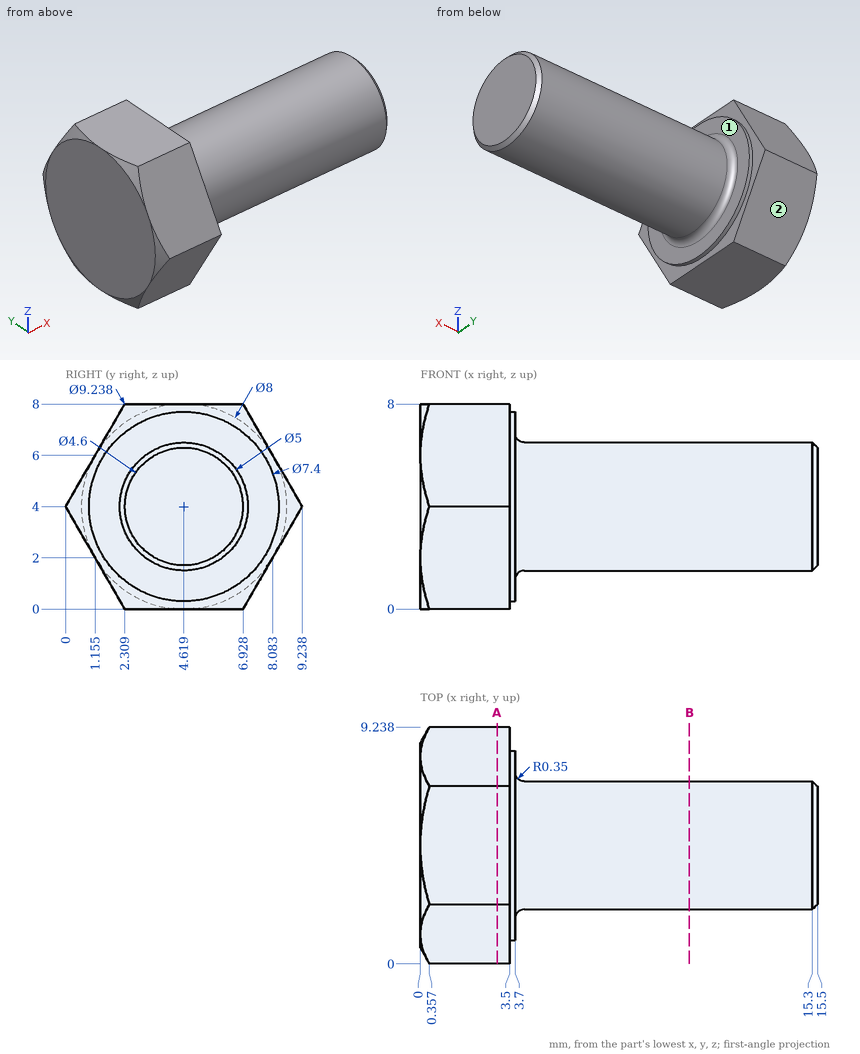
Job drawing, mm, ordinate dimensions from the low corner. One solid piece. A direction names the side the tool comes from. Coordinates: 2 decimals unless noted, no trailing zeros. Order: outer loops, then holes, each group sorted by start corner. A loop starts at its lowest first (then second) coordinate and runs counter-clockwise, first axis right, second up. Notation, with made-up numbers: (81.5, 27) -> (109.5, 27) arc R33 cw to (109.5, 66) -> close; hole circle Ø8 at (82, 55). An arc over 180 degrees is marked (long way). Answer in a Markdown table with one row per item. Add a question column.
Q1. Band-saw the part on A-A, the plane x = 3. List the corners of the cut face in (y, z).
Q2. Which spindle directions (+Z, -Z, +X, -X, +Y, -Y) get a long thin tool onto all of the face, cutting with end or side? Do the marked faces 1 and 2. Say none if no direction does.
Q3. Wall check: line 1 along X through (y, z) = (2, 2.5); line 2 along Z through (x, y) = (10, 4); line 3 along Y through (x, z) = (8, 6). Give the ranges that are in metal, low to high. Write a range as [from, to].
Q4. Drop flat-ended pins along their axis: pin 1 (1 mm diameter, centred on x = 9.5, y = 4, fed in from +Z); pin 2 (1.5 mm diameter, centred on x = 5, z = 5, fed in from -Y); pin 3 (2 mm diameter, centred on y = 7, z = 6.5, fed in from +X). Give the stop position or say it passes through.
Q5. Band-saw the part on B-B, the plane x = 10.5. List the corners of the cut face in (y, z), then the cut area to 3 significant figures.
Answers follow:
| question | item | result |
|---|---|---|
| 1 | outline | (0, 4) -> (2.31, 0) -> (6.93, 0) -> (9.24, 4) -> (6.93, 8) -> (2.31, 8) -> close |
| 2 | face 1 | +X |
| 2 | face 2 | -Z, +X, -X, +Y |
| 3 | line 1 | [0, 3.7] |
| 3 | line 2 | [1.58, 6.42] |
| 3 | line 3 | [3.12, 6.12] |
| 4 | pin 1 | z = 6.5 |
| 4 | pin 2 | y = 2.13 |
| 4 | pin 3 | x = 15.35 |
| 5 | outline | circle Ø5 at (4.62, 4) |
| 5 | area | 19.6 mm^2 |
